```python
from build123d import *

# Parameters (mm, degrees)
EXTRUDE_1_DEPTH          = 2
EXTRUDE_1_DEPTH_BACK     = 1
SKETCH_1_W               = 45
SKETCH_1_H               = 15
SKETCH_2_W               = 45
SKETCH_2_H               = 3.5
EXTRUDE_2_DEPTH          = 50
SKETCH_3_R               = 1.55
CUT_EXTRUDE_1_DEPTH      = 69.92024376
SKETCH_4_R               = 1.55
CUT_EXTRUDE_2_DEPTH      = 71.384657419
SKETCH_5_W               = 31
SKETCH_5_H               = 5
EXTRUDE_4_DEPTH          = 10
SKETCH_8_W               = 7
SKETCH_8_H               = 40
CUT_EXTRUDE_5_DEPTH      = 10
FILLET_4_RADIUS          = 5
FILLET_4_LENGTH          = 3.5
FILLET_5_RADIUS          = 5
FILLET_5_LENGTH          = 3.5
CUT_EXTRUDE_7_DEPTH      = 67.128662469
CUT_EXTRUDE_7_DEPTH_BACK = 67.128662469
EXTRUDE_5_DEPTH          = 31
FILLET_6_R               = 5


with BuildPart() as part:
    # 草图1 → 凸台-拉伸1 (new, two sides: drawn at the far end of the back side and taken through both)
    with BuildSketch(Plane(origin=(0, 0, 0), x_dir=(1, 0, 0), z_dir=(0, 1, 0)).offset(-EXTRUDE_1_DEPTH_BACK)):
        with Locations((22.5, -7.5)):
            Rectangle(SKETCH_1_W, SKETCH_1_H)
    extrude(amount=EXTRUDE_1_DEPTH + EXTRUDE_1_DEPTH_BACK)

    # 草图2 → 凸台-拉伸2 (add)
    with BuildSketch(Plane(origin=(0, 2, 0), x_dir=(1, 0, 0), z_dir=(0, 1, 0))):
        with Locations((22.5, -1.75)):
            Rectangle(SKETCH_2_W, SKETCH_2_H)
    extrude(amount=EXTRUDE_2_DEPTH)

    # 草图3 → 切除-拉伸1 (cut, through all)
    with BuildSketch(Plane(origin=(0, 2, 0), x_dir=(1, 0, 0), z_dir=(0, 1, 0))):
        with Locations(Location((8, -10, 0), (0, 0, 270))):
            Circle(SKETCH_3_R)
        with Locations(Location((37, -10, 0), (0, 0, 270))):
            Circle(SKETCH_3_R)
    extrude(amount=-CUT_EXTRUDE_1_DEPTH, mode=Mode.SUBTRACT)

    # 草图4 → 切除-拉伸2 (cut, through all)
    with BuildSketch(Plane(origin=(0, 0, 0), x_dir=(-1, 0, 0), z_dir=(0, 0, -1))):
        with Locations((-39.5, 47)):
            Circle(SKETCH_4_R)
        with Locations((-5.5, 47)):
            Circle(SKETCH_4_R)
    extrude(amount=-CUT_EXTRUDE_2_DEPTH, mode=Mode.SUBTRACT)

    # 草图5 → 凸台-拉伸4 (add)
    with BuildSketch(Plane(origin=(0, 0, 0), x_dir=(-1, 0, 0), z_dir=(0, 0, -1))):
        with Locations((-22.5, 39.5)):
            Rectangle(SKETCH_5_W, SKETCH_5_H)
    extrude(amount=EXTRUDE_4_DEPTH)

    # 草图8 → 切除-拉伸5 (cut)
    with BuildSketch(Plane(origin=(0, 0, 0), x_dir=(-1, 0, 0), z_dir=(0, 0, -1))):
        with Locations((-41.5, 22)):
            Rectangle(SKETCH_8_W, SKETCH_8_H)
        with Locations((-3.5, 22)):
            Rectangle(SKETCH_8_W, SKETCH_8_H)
    extrude(amount=-CUT_EXTRUDE_5_DEPTH, mode=Mode.SUBTRACT)

    # 圆角4: full round fillet: the end face becomes a half cylinder, R = half its width
    fillet_4_face = Plane((45, 47, 1.75), x_dir=(0, 0, 1), z_dir=(1, 0, 0))  # on the end face: x along it, z out of the body
    fillet_4_slab = fillet_4_face.offset(-FILLET_4_RADIUS / 2) * Box(FILLET_4_LENGTH, 2 * FILLET_4_RADIUS, FILLET_4_RADIUS, mode=Mode.PRIVATE)  # the body's end, R deep
    fillet_4_round = Plane((40, 47, 1.75), x_dir=(1, 0, 0), z_dir=(0, 0, 1)) * Cylinder(FILLET_4_RADIUS, FILLET_4_LENGTH, mode=Mode.PRIVATE)  # its axis R under the face
    add(fillet_4_slab - fillet_4_round, mode=Mode.SUBTRACT)

    # 圆角5: full round fillet: the end face becomes a half cylinder, R = half its width
    fillet_5_face = Plane((0, 47, 1.75), x_dir=(0, 0, -1), z_dir=(-1, 0, 0))  # on the end face: x along it, z out of the body
    fillet_5_slab = fillet_5_face.offset(-FILLET_5_RADIUS / 2) * Box(FILLET_5_LENGTH, 2 * FILLET_5_RADIUS, FILLET_5_RADIUS, mode=Mode.PRIVATE)  # the body's end, R deep
    fillet_5_round = Plane((5, 47, 1.75), x_dir=(-1, 0, 0), z_dir=(0, 0, -1)) * Cylinder(FILLET_5_RADIUS, FILLET_5_LENGTH, mode=Mode.PRIVATE)  # its axis R under the face
    add(fillet_5_slab - fillet_5_round, mode=Mode.SUBTRACT)

    # 草图18 → 切除-拉伸7 (cut, two sides: drawn at the far end of the back side and taken through both)
    with BuildSketch(Plane.ZY.offset(-7).offset(-CUT_EXTRUDE_7_DEPTH_BACK)):
        Polygon((0, 37), (0, 42.006951797), (-10, 42), (-10, 37), align=None)
    extrude(amount=CUT_EXTRUDE_7_DEPTH + CUT_EXTRUDE_7_DEPTH_BACK, mode=Mode.SUBTRACT)

    # 草图20 → 凸台-拉伸5 (add)
    with BuildSketch(Plane.ZY.offset(-7)):
        Polygon((3.5, 42), (6, 2), (3.5, 2), align=None)
    extrude(amount=-EXTRUDE_5_DEPTH)

    # 圆角6
    fillet_6_edges = [part.edges().sort_by_distance(p)[0] for p in [
        (0, 0.5, 0),
        (45, 0.5, 0),
        (45, 0.5, 15),
        (0, 0.5, 15),
    ]]
    fillet(fillet_6_edges, radius=FILLET_6_R)


solid = part.part
```
Input: part model. Units: mm. Frame: model coordinates. A direction names the side the tool comes from. Give positions to 0.01 mm unless a question says otherwise; leave off trailing zeros. Order: outer loops, then holes, each group sorted by start corner. A loop starts at its lowest first (then second) coordinate and runs counter-clockwise, first axis right, second up. Notation, with made-up numbers: M 46,-37 L 60,-37 A17 ccw 60,-14 Z; hole C 75.5,-29.5 d10. An arc over 180 degrees is marked long. One line per question, with ' | ' between items. Start each with the question number.
1. First-contact query: pin 1 Ø4 at (x, z) = (8, 10) entering from -Y; pin 2 Ø3 at (x, z) = (36, 11) entering from +Y; pin 3 Ø2.5 at (x, y) = (5.5, 47) entering from +Z; pin 4 Ø3 at (x, y) = (20.5, 46) entering from +Z. Flat tips, straight axial feed; report the tip coordinate or a pass-through.
2. Pull-direction query (Y, two-part tool) for faces 1 (the face through (7, 22, 2)), 2 (the face through (35.487, 0.521, 9.664)), 3 (the face through (22, 52, 2)), 4 (the face through (22, -1, 7)); classes: released by +Y, released by -Y, zero draft, split by the parting line, or undercut.
3. Access query for faces 5 (the face through (2, 0, 1)), 6 (the face through (39, 42, 2)), 7 (the face through (43, 0, 1)). Directions: +Z, -Z, +X, -X, +Y, -Y. A direction counts if a zero-diameter tool reaches every point of the face in a straight line with its end or side. Return the directions, or none.
4. Material intervals for probe 1 along Y at (x, z) = (5.5, 2.45); probe 2 along Z at (x, y) = (37, 1.3); probe 3 along X at (y, z) = (46, 2), sorted ascending. Write a range as [from, to].
5. Section query C-C (x = 22.5). Return the cut outline in (y, z).
6. Section query B-B (x = 37). Return the cut outline in (y, z), and give its area (3 significant figures).
7. Section query A-A (y = 47). Return the cut outline in (x, z), and give its area (3 significant figures).
8. Section query D-D (y = 6). Return the cut outline in (x, z), and give its area (3 significant figures).
Here are the results:
1) pin 1: y = -1 | pin 2: y = 2 | pin 3: through | pin 4: z = 3.5
2) face 1: undercut | face 2: zero draft | face 3: released by +Y | face 4: released by -Y
3) face 5: -Z, -X, -Y | face 6: +Z, -Z, +X | face 7: -Z, +X, -Y
4) probe 1: [-1, 2], [42, 45.45], [48.55, 52] | probe 2: [0, 8.45], [11.55, 15] | probe 3: [0.1, 4.32], [6.68, 38.32], [40.68, 44.9]
5) outline: M -1,0 L 52,0 L 52,3.5 L 42,3.5 L 2,6 L 2,15 L -1,15 Z
6) outline: M -1,0 L 52,0 L 52,3.5 L 42,3.5 L 2,6 L 2,8.45 L -1,8.45 Z; M -1,11.55 L 2,11.55 L 2,15 L -1,15 Z | area: 261 mm²
7) outline: M 0,0 L 3.95,0 L 3.95,3.5 L 0,3.5 Z; M 7.05,0 L 37.95,0 L 37.95,3.5 L 7.05,3.5 Z; M 41.05,0 L 45,0 L 45,3.5 L 41.05,3.5 Z | area: 136 mm²
8) outline: M 7,0 L 38,0 L 38,5.75 L 7,5.75 Z | area: 178 mm²
